from build123d import *

# Parameters (mm, degrees)
F0_W          = 65
F0_H          = 60
F0_W_2        = 6.15
F0_H_2        = 13.25
F1_DEPTH      = 15
F3_DEPTH      = 14
F5_DEPTH      = 4
F6_R          = 3
F7_DEPTH      = 8
F9_DEPTH      = 90
F10_T4_DEPTH  = 29.425
F10_S5_R      = 16.5
F10_T6_DEPTH  = 16
F10_T10_DEPTH = 44.425
F10_S11_R     = 16.5
F10_T12_DEPTH = 24
F10_T17_DEPTH = 44.425
F10_S18_R     = 16.5
F10_T19_DEPTH = 24
F10_T24_DEPTH = 29.425
F10_S25_R     = 16.5
F10_T26_DEPTH = 16
F10_T30_DEPTH = 44.425
F10_S31_R     = 16.5
F10_T32_DEPTH = 24
F10_T37_DEPTH = 29.425
F10_S38_R     = 16.5
F10_T39_DEPTH = 16
F10_T43_DEPTH = 29.425
F10_S44_R     = 16.5
F10_T45_DEPTH = 16
F10_T49_DEPTH = 44.425
F10_S50_R     = 16.5
F10_T51_DEPTH = 24
F11_T1_DEPTH  = 80.4300979278
F11_T3_DEPTH  = 51.7830754439
F11_T5_DEPTH  = 51.7830754439
F11_T7_DEPTH  = 31.4300979278
F11_T9_DEPTH  = 31.4300979278


# Not quite as in the source:
# - a fillet or chamfer that OpenCascade refuses, or shapes differently, is made with other operations: its cross-section is extruded or revolved along the edge and cut away or added


with BuildPart() as f1:
    # F0 (on Top) → F1 (new body)
    with BuildSketch(Plane.XY):
        Rectangle(F0_W, F0_H)
        with Locations((0, 6.625)):
            Rectangle(F0_W_2, F0_H_2, mode=Mode.SUBTRACT)
    extrude(amount=F1_DEPTH)

    # F2 (on Front) → F3 (join, symmetric)
    with BuildSketch(Plane.XZ):
        with BuildLine():
            Line((-3.075, 0), (-32.5, 0))
            Line((-32.5, 0), (-32.5, -38.5))
            Line((-32.5, -38.5), (-16.5, -38.5))
            Line((-16.5, -38.5), (-16.5, -16.5))
            ThreePointArc((-16.5, -16.5), (-12.7080191218, -5.9759204678), (-3.075, -0.2890661898))
            Line((-3.075, -0.2890661898), (-3.075, 0))
        make_face()
        with BuildLine():
            Line((3.075, 0), (3.075, -0.2890661898))
            ThreePointArc((3.075, -0.2890661898), (12.7080191218, -5.9759204678), (16.5, -16.5))
            Line((16.5, -16.5), (16.5, -38.5))
            Line((16.5, -38.5), (32.5, -38.5))
            Line((32.5, -38.5), (32.5, 0))
            Line((32.5, 0), (3.075, 0))
        make_face()
    extrude(amount=F3_DEPTH, both=True)

    # F4 (on face) → F5 (cut)
    with BuildSketch(Plane.XY.offset(15)):
        with BuildLine():
            ThreePointArc((12, -21.9317121995), (25, 0), (12, 21.9317121995))
            Line((12, 21.9317121995), (12, 35))
            Line((12, 35), (-12, 35))
            Line((-12, 35), (-12, 21.9317121995))
            ThreePointArc((-12, 21.9317121995), (-25, 0), (-12, -21.9317121995))
            Line((-12, -21.9317121995), (-12, -35))
            Line((-12, -35), (12, -35))
            Line((12, -35), (12, -21.9317121995))
        make_face()
    extrude(amount=-F5_DEPTH, mode=Mode.SUBTRACT)

    # F6 (on face) → F7 (cut)
    with BuildSketch(Plane.XY.offset(11)):
        with Locations((-12.7, 12.7)):
            Circle(F6_R)
        with Locations((12.3, 12.7)):
            Circle(F6_R)
        with Locations((12.3, -12.3)):
            Circle(F6_R)
        with Locations((-12.7, -12.3)):
            Circle(F6_R)
    extrude(amount=-F7_DEPTH, mode=Mode.SUBTRACT)

    # F8 (on face) → F9 (cut)
    with BuildSketch(Plane.YZ.offset(32.5)):
        with BuildLine():
            Line((0, -15.3778724497), (0, 0))
            Line((0, 0), (-14, 0))
            Line((-14, 0), (-14, -38.5))
            ThreePointArc((-14, -38.5), (-5.2228777507, -28.0149492966), (0, -15.3778724497))
        make_face()
    extrude(amount=-F9_DEPTH, mode=Mode.SUBTRACT)

    # F10: fillet of radius 3 on 4 edges, made by hand


with BuildPart() as f10_tool2:
    # F10_s3 → F10_t4 (new body)
    with BuildSketch(Plane.YZ.offset(32.5)):
        with BuildLine():
            ThreePointArc((0, -3), (-0.8786796564, -0.8786796564), (-3, 0))
            Line((-3, 0), (0, 0))
            Line((0, 0), (0, -3))
        make_face()
    extrude(amount=-F10_T4_DEPTH)

    # F10_s5 → F10_t6 (cut, symmetric)
    with BuildSketch(Plane.XZ.offset(1.5)):
        with Locations((0, -16.5)):
            Circle(F10_S5_R)
    extrude(amount=F10_T6_DEPTH, both=True, mode=Mode.SUBTRACT)


with BuildPart() as f1_1:
    add(f1.part)

    # F10_t1: union F10_tool2
    add(f10_tool2.part)


with BuildPart() as f10_tool8:
    # F10_s9 → F10_t10 (new body)
    with BuildSketch(Plane.YZ.offset(40)):
        with BuildLine():
            ThreePointArc((0, -3), (-0.8786796564, -0.8786796564), (-3, 0))
            Line((-3, 0), (0, 0))
            Line((0, 0), (0, -3))
        make_face()
    extrude(amount=-F10_T10_DEPTH)

    # F10_s11 → F10_t12 (cut, symmetric)
    with BuildSketch(Plane.XZ.offset(1.5)):
        with Locations((0, -16.5)):
            Circle(F10_S11_R)
    extrude(amount=F10_T12_DEPTH, both=True, mode=Mode.SUBTRACT)

    split(bisect_by=Plane.YZ.offset(-3.075), keep=Keep.BOTTOM)


with BuildPart() as f1_2:
    add(f1_1.part)

    # F10_t7: union F10_tool8
    add(f10_tool8.part)


with BuildPart() as f10_tool15:
    # F10_s16 → F10_t17 (new body)
    with BuildSketch(Plane.YZ.offset(4.425)):
        with BuildLine():
            ThreePointArc((0, -3), (-0.8786796564, -0.8786796564), (-3, 0))
            Line((-3, 0), (0, 0))
            Line((0, 0), (0, -3))
        make_face()
    extrude(amount=-F10_T17_DEPTH)

    # F10_s18 → F10_t19 (cut, symmetric)
    with BuildSketch(Plane.XZ.offset(1.5)):
        with Locations((0, -16.5)):
            Circle(F10_S18_R)
    extrude(amount=F10_T19_DEPTH, both=True, mode=Mode.SUBTRACT)

    split(bisect_by=Plane.YZ.offset(3.075), keep=Keep.TOP)


with BuildPart() as f1_3:
    add(f1_2.part)

    # F10_t14: union F10_tool15
    add(f10_tool15.part)


with BuildPart() as f10_tool22:
    # F10_s23 → F10_t24 (new body)
    with BuildSketch(Plane.YZ.offset(-3.075)):
        with BuildLine():
            ThreePointArc((0, -3), (-0.8786796564, -0.8786796564), (-3, 0))
            Line((-3, 0), (0, 0))
            Line((0, 0), (0, -3))
        make_face()
    extrude(amount=-F10_T24_DEPTH)

    # F10_s25 → F10_t26 (cut, symmetric)
    with BuildSketch(Plane.XZ.offset(1.5)):
        with Locations((0, -16.5)):
            Circle(F10_S25_R)
    extrude(amount=F10_T26_DEPTH, both=True, mode=Mode.SUBTRACT)


with BuildPart() as f1_4:
    add(f1_3.part)

    # F10_t21: union F10_tool22
    add(f10_tool22.part)


with BuildPart() as f10_tool28:
    # F10_s29 → F10_t30 (new body)
    with BuildSketch(Plane.YZ.offset(4.425)):
        with BuildLine():
            ThreePointArc((14, -3), (14.8786796564, -0.8786796564), (17, 0))
            Line((17, 0), (14, 0))
            Line((14, 0), (14, -3))
        make_face()
    extrude(amount=-F10_T30_DEPTH)

    # F10_s31 → F10_t32 (cut, symmetric)
    with BuildSketch(Plane.XZ.offset(-15.5)):
        with Locations((0, -16.5)):
            Circle(F10_S31_R)
    extrude(amount=F10_T32_DEPTH, both=True, mode=Mode.SUBTRACT)

    split(bisect_by=Plane.YZ.offset(3.075), keep=Keep.TOP)


with BuildPart() as f1_5:
    add(f1_4.part)

    # F10_t27: union F10_tool28
    add(f10_tool28.part)


with BuildPart() as f10_tool35:
    # F10_s36 → F10_t37 (new body)
    with BuildSketch(Plane.YZ.offset(-3.075)):
        with BuildLine():
            ThreePointArc((14, -3), (14.8786796564, -0.8786796564), (17, 0))
            Line((17, 0), (14, 0))
            Line((14, 0), (14, -3))
        make_face()
    extrude(amount=-F10_T37_DEPTH)

    # F10_s38 → F10_t39 (cut, symmetric)
    with BuildSketch(Plane.XZ.offset(-15.5)):
        with Locations((0, -16.5)):
            Circle(F10_S38_R)
    extrude(amount=F10_T39_DEPTH, both=True, mode=Mode.SUBTRACT)


with BuildPart() as f1_6:
    add(f1_5.part)

    # F10_t34: union F10_tool35
    add(f10_tool35.part)


with BuildPart() as f10_tool41:
    # F10_s42 → F10_t43 (new body)
    with BuildSketch(Plane.YZ.offset(32.5)):
        with BuildLine():
            ThreePointArc((14, -3), (14.8786796564, -0.8786796564), (17, 0))
            Line((17, 0), (14, 0))
            Line((14, 0), (14, -3))
        make_face()
    extrude(amount=-F10_T43_DEPTH)

    # F10_s44 → F10_t45 (cut, symmetric)
    with BuildSketch(Plane.XZ.offset(-15.5)):
        with Locations((0, -16.5)):
            Circle(F10_S44_R)
    extrude(amount=F10_T45_DEPTH, both=True, mode=Mode.SUBTRACT)


with BuildPart() as f1_7:
    add(f1_6.part)

    # F10_t40: union F10_tool41
    add(f10_tool41.part)


with BuildPart() as f10_tool47:
    # F10_s48 → F10_t49 (new body)
    with BuildSketch(Plane.YZ.offset(40)):
        with BuildLine():
            ThreePointArc((14, -3), (14.8786796564, -0.8786796564), (17, 0))
            Line((17, 0), (14, 0))
            Line((14, 0), (14, -3))
        make_face()
    extrude(amount=-F10_T49_DEPTH)

    # F10_s50 → F10_t51 (cut, symmetric)
    with BuildSketch(Plane.XZ.offset(-15.5)):
        with Locations((0, -16.5)):
            Circle(F10_S50_R)
    extrude(amount=F10_T51_DEPTH, both=True, mode=Mode.SUBTRACT)

    split(bisect_by=Plane.YZ.offset(-3.075), keep=Keep.BOTTOM)


with BuildPart() as f1_8:
    add(f1_7.part)

    # F10_t46: union F10_tool47
    add(f10_tool47.part)

    # F11: chamfer of 3 on 6 edges, made by hand

    # F11_s2 → F11_t1 (cut)
    with BuildSketch(Plane.YZ.offset(-40.2150489639)):
        Polygon((-30, 3), (-27, 0), (-30, 0), align=None)
        Polygon((27, 0), (30, 3), (30, 0), align=None)
    extrude(amount=F11_T1_DEPTH, mode=Mode.SUBTRACT)

    # F11_s4 → F11_t3 (cut)
    with BuildSketch(Plane.YZ.offset(-50.391537722)):
        with BuildLine():
            Line((-6.8950157601, -38.5), (-9.1963693219, -33.5754814152))
            ThreePointArc((-9.1963693219, -33.5754814152), (-11.4890994339, -36.1144458386), (-14, -38.5))
            Line((-14, -38.5), (-6.8950157601, -38.5))
        make_face()
    extrude(amount=F11_T3_DEPTH, mode=Mode.SUBTRACT)

    # F11_s6 → F11_t5 (cut)
    with BuildSketch(Plane.YZ.offset(-1.391537722)):
        with BuildLine():
            Line((-9.1963693219, -33.5754814152), (-6.8950157601, -38.5))
            Line((-6.8950157601, -38.5), (-14, -38.5))
            ThreePointArc((-14, -38.5), (-11.4890994339, -36.1144458386), (-9.1963693219, -33.5754814152))
        make_face()
    extrude(amount=F11_T5_DEPTH, mode=Mode.SUBTRACT)

    # F11_s8 → F11_t7 (cut)
    with BuildSketch(Plane.YZ.offset(8.7849510361)):
        Polygon((11, -38.5), (14, -35.5), (14, -38.5), align=None)
    extrude(amount=F11_T7_DEPTH, mode=Mode.SUBTRACT)

    # F11_s10 → F11_t9 (cut)
    with BuildSketch(Plane.YZ.offset(-40.2150489639)):
        Polygon((11, -38.5), (14, -35.5), (14, -38.5), align=None)
    extrude(amount=F11_T9_DEPTH, mode=Mode.SUBTRACT)


solid = f1_8.part
Geometry check sheet. Reference: the model listing, model coordinates, mm. A direction names the side the tool comes from. Round coordinates to 2 decimals unless told otherwise and drop trailing zeros. Loops run counter-clockwise (first coordinate to the right, second up) from the corner with the lowest first, then second, coordinate; pieces in that order, holes last. Notation, with made-up numbers: (78, 68.5) - (114, 68.5) arc R8 ccw to (114, 76.5) - close; hole circle Ø3 at (-25.5, 70.5). An arc over 180 degrees is marked (long way). Answer as CSV lines item,"result".
(1) Release check for a two-part mould opening along Y. For faces 6 (the face through (25, 0, 13)), 7 (the face through (17.99, 14.86, -0.9)), 8 (the face through (0, -13, 0)) record: released by +Y, released by -Y, zero draft, split by the parting line, or undercut.
Output values:
face 6,"undercut"
face 7,"released by +Y"
face 8,"zero draft"
(2) Cross-section at C-C, the plane z = 8. Enter the section's corners in (x, y) (3 decimals), and give its area (3 significant figures).
Output values:
outline,"(-32.5, -30) - (32.5, -30) - (32.5, 30) - (-32.5, 30) - close; hole circle Ø6 at (-12.7, -12.3); hole circle Ø6 at (-12.7, 12.7); hole (-3.075, 0) - (3.075, 0) - (3.075, 13.25) - (-3.075, 13.25) - close; hole circle Ø6 at (12.3, -12.3); hole circle Ø6 at (12.3, 12.7)"
area,"3,710 mm²"
(3) Cross-section at B-B, the plane y = 6.5. Enter the section's corners in (x, z) (3 decimals).
Output values:
outline,"(-32.5, -38.5) - (-16.5, -38.5) - (-16.5, -16.5) arc R16.5 cw to (-3.075, -0.289) - (-3.075, 11) - (-24.14, 11) - (-24.14, 15) - (-32.5, 15) - close; (3.075, -0.289) arc R16.5 cw to (16.5, -16.5) - (16.5, -38.5) - (32.5, -38.5) - (32.5, 15) - (24.14, 15) - (24.14, 11) - (3.075, 11) - close"
(4) Material ranges on line 1 along Y through (x, z) = (-12.7, 9.5); line 2 along X through (y, z) = (5.5, -18); line 3 along X through (y, z) = (10, 7.5) (3 decimals), recorded low to high.
Output values:
line 1,"y = -30 to -15.3, -9.3 to 9.7, 15.7 to 30"
line 2,"x = -32.5 to -16.5, 16.5 to 32.5"
line 3,"x = -32.5 to -14.008, -11.392 to -3.075, 3.075 to 10.992, 13.608 to 32.5"
(5) Cross-section at D-D, the plane x = 26. Enter the section's corners in (y, z).
Output values:
outline,"(-30, 3) - (-27, 0) - (-3, 0) arc R3 cw to (0, -3) - (0, -15.38) arc R45 cw to (-9.2, -33.58) - (-6.9, -38.5) - (11, -38.5) - (14, -35.5) - (14, -3) arc R3 cw to (17, 0) - (27, 0) - (30, 3) - (30, 15) - (-30, 15) - close"
(6) Cross-section at A-A, the plane x = -1.5. Enter the section's corners in (y, z), and give its area (3 significant figures).
Output values:
outline,"(-30, 3) - (-27, 0) - (0, 0) - (0, 11) - (-30, 11) - close; (13.25, 0) - (27, 0) - (30, 3) - (30, 11) - (13.25, 11) - close"
area,"505 mm²"
(7) Depth check by flat-ended pin: pin 1 Ø6.5 at (x, y) = (-13.5, -12) entering from +Z; pin 2 Ø18.5 at (x, z) = (-17.5, -22) entering from +Y; pin 3 Ø10 at (x, z) = (-18.5, -12) entering from -Y. Enter the tip coordinate at first touch or a pass-through.
Output values:
pin 1,"stops at z = 11"
pin 2,"stops at y = 14"
pin 3,"stops at y = -0.43"
(8) Set-up check for faces 1 (the face through (15.07, -13.45, 7.06)), 2 (the face through (0, 0, 5)), 3 (the face through (-24.369, -3.619, -25.133)), 4 (the face through (12, 26, 13)), 5 (the face through (16.5, 5, -27)): record each of +Z, -Z, +X, -X, +Y, -Y from which the full face is reachable in a straight line by a thin tool's end or side.
Output values:
face 1,"+Z"
face 2,"+Z, -Z"
face 3,"+X, -X, -Y"
face 4,"+Z, +Y, -Y"
face 5,"-Z, +Y, -Y"
